Build history of the part. All positions in model axes, mm. A direction names the side the tool comes from. Give positions to 0.01 mm unless a question says otherwise; leave off trailing zeros. Write each loop counter-clockwise with the first axis right and the second up, starting at its lowest first coordinate (ties: lowest second). Pieces come first, ordered by that corner, then holes. Notation, with made-up numbers: M -30.75,-24 L -0.75,-24 A25 cw -0.75,12 Z; hole C 9,64.5 d6. An arc over 180 degrees is marked long. Return JSON: item names as keys, results as strings. Group by question number.
Q1. Band-saw the part on A-A, the plane y = 0. Give the cut face in (x, z).
Q2. Band-saw the part on C-C, the plane z = 9. Give the cut face in (x, y).
Q3. Flat gauge pins, fed straight in: pin 1 Ø3 at (x, y) = (2, 4) entering from -Z; pin 2 Ø1.1 at (x, z) = (0, 31) entering from +Y; pin 3 Ø1 at (x, y) = (2.5, -1) entering from +Z. Where does each tip first touch, or does it go through?
Q4. Band-saw the part on B-B, the plane x = 0.75. Give the cut face in (y, z).
Q5. Wall check: probe 1 along Z at (x, y) = (-2.25, -2.5); probe 2 along Z at (x, y) = (0.5, 1.25); probe 3 along Y at (x, z) = (-0.25, 14.5). Give the ranges that are in metal, low to high.
Q6. Band-saw the part on D-D, the plane y = -4.25. Give the cut face in (x, z).
Q7. Tool access for faces 1 (the flat face through (4, -5, 15)), 2 (the flat face through (0, 1, 29)), 3 (the flat face through (-4, -5, 15)): list every direction of +Z, -Z, +X, -X, +Y, -Y with a clear straight run to the whole face (end or side of a thin tool).
Autodesk Fusion 360 part; units mm, degrees
sketch "Sketch1" plane through (0, 0, 0) normal (0, 0, 1) x (1, 0, 0)
  circle A0 centre (0, 0) radius 6
  line L0 (5, -7) -> (-5, -7)
  line L1 (-5, -7) -> (-5, 7)
  line L2 (-5, 7) -> (5, 7)
  line L3 (5, 7) -> (5, -7)
  line L4 (5, -7) -> (-5, 7) construction
  line L5 (-5, -7) -> (5, 7) construction
  dimension "d1" = 12
extrude "Extrude1" add sketch "Sketch1" along normal blind 15 contours A0 L1 L3
sketch "Sketch2" plane through (0, 0, 0) normal (0, 0, 1) x (1, 0, 0)
  line L0 (5, -6) -> (-5, -6)
  line L1 (-5, -6) -> (-5, 6)
  line L2 (-5, 6) -> (5, 6)
  line L3 (5, 6) -> (5, -6)
  line L4 (5, -6) -> (-5, 6) construction
  line L5 (-5, -6) -> (5, 6) construction
sketch "Sketch3" plane through (0, 0, 0) normal (0, 0, 1) x (1, 0, 0)
sketch "Sketch4" plane through (0, 0, 0) normal (0, 0, 1) x (1, 0, 0)
sketch "Sketch5" plane through (0, 0, 15) normal (0, 0, 1) x (-1, 0, 0)
  arc A0 (5, 3.3166) -> (-5, 3.3166) centre (0, 0) ccw
  line L0 (-5, 3.3166) -> (-5, -3.3166)
  arc A1 (-5, -3.3166) -> (5, -3.3166) centre (0, 0) ccw
  line L1 (5, -3.3166) -> (5, 3.3166)
  line L2 (-5, 6) -> (5, 6)
  line L3 (5, 6) -> (5, -6)
  line L4 (5, -6) -> (-5, -6)
  line L5 (-5, -6) -> (-5, 6)
  line L6 (-5, 6) -> (5, -6) construction
  line L7 (5, 6) -> (-5, -6) construction
extrude "Extrude2" add sketch "Sketch5" along normal blind 9
sketch "Sketch6" plane through (0, 0, 24) normal (0, 0, 1) x (-1, 0, 0)
  line L0 (-5, -6) -> (5, -6)
  line L1 (5, -6) -> (5, 6)
  line L2 (5, 6) -> (-5, 6)
  line L3 (-5, 6) -> (-5, -6)
  circle A0 centre (0, 0) radius 1.5
  line L4 (0, 0) -> (0, -1)
  line L5 (0, -1) -> (-1.118, -1)
  line L6 (0, -1) -> (1.118, -1)
  line L7 (1.118, -1) -> (-1.118, -1)
  dimension "d6" = 3
extrude "Extrude3" add sketch "Sketch6" along normal blind 9 contours A0 L5 L6 L7 picked at (0.0074, 0.6639)
extrude "Extrude5" add sketch "Sketch6" along normal blind 2 contours A0 L5 L6 L7 picked at (0.0699, -1.3284)
extrude "Extrude4" [suppressed]
From the geometry:
{
 "1": {"outline": "M -5,0 L 5,0 L 5,24 L 1.5,24 L 1.5,33 L -1.5,33 L -1.5,24 L -5,24 Z"},
 "2": {"outline": "M -5,-3.32 A6 ccw 5,-3.32 L 5,3.32 A6 ccw -5,3.32 Z"},
 "3": {"pin 1": "stops at z = 0", "pin 2": "stops at y = 1", "pin 3": "stops at z = 24"},
 "4": {"outline": "M -6,15 L -5.95,15 L -5.95,0 L 5.95,0 L 5.95,15 L 6,15 L 6,24 L 1.3,24 L 1.3,26 L 1,26 L 1,33 L -1.3,33 L -1.3,24 L -6,24 Z"},
 "5": {"probe 1": "z = 0 to 24", "probe 2": "z = 0 to 26", "probe 3": "y = -5.99 to 5.99"},
 "6": {"outline": "M -5,15 L -4.24,15 L -4.24,0 L 4.24,0 L 4.24,15 L 5,15 L 5,24 L -5,24 Z"},
 "7": {"face 1": "-Z, +X, -Y", "face 2": "+Z, +X, -X, +Y", "face 3": "-Z, -X, -Y"}
}
